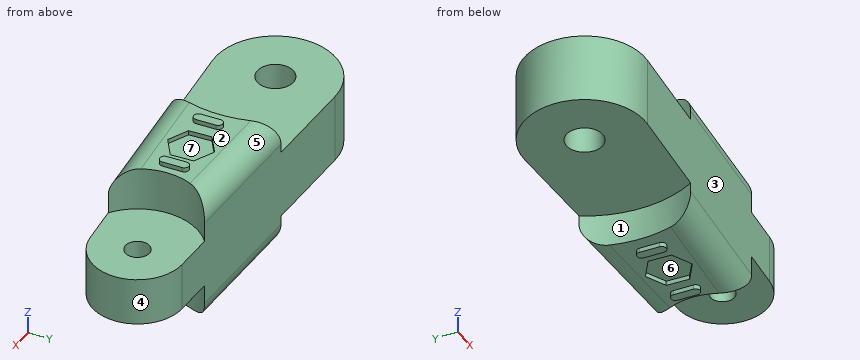
```python
from build123d import *

# Parameters (mm, degrees)
BOSS_EXTRUDE1_DEPTH    = 22.5
SKETCH2_R              = 37.5
SKETCH2_R_2            = 20
CUT_EXTRUDE1_DEPTH     = 11
FILLET1_R              = 8
SKETCH4_R              = 6
SKETCH4_R_2            = 4
CUT_EXTRUDE2_DEPTH     = 40
CUT_EXTRUDE3_DEPTH     = 1.5
BOSS_EXTRUDE2_DEPTH    = 1.5
SKETCH7_R              = 20
CUT_EXTRUDE4_DEPTH     = 3.5
BODY_MOVE_COPY7_ANGLE  = 178.232303169
BODY_MOVE_COPY8_ANGLE  = 1.26
BODY_MOVE_COPY9_ANGLE  = 1.26
BODY_MOVE_COPY10_ANGLE = 180


with BuildPart() as part:
    # Sketch1 → Boss-Extrude1 (new body, symmetric)
    with BuildSketch(Plane(origin=(0, 0, 0), x_dir=(1, 0, 0), z_dir=(0, 1, 0))):
        with BuildLine():
            Line((-91.135271219, -13.013928685), (-1.541618241, -19.940496814))
            ThreePointArc((-1.541618241, -19.940496814), (19.99534612, -0.431431984), (-0.680086883, 19.988433701))
            Line((-0.680086883, 19.988433701), (-90.489122701, 16.932769202))
            ThreePointArc((-90.489122701, 16.932769202), (-104.975567128, 2.265017913), (-91.135271219, -13.013928685))
        make_face()
    extrude(amount=BOSS_EXTRUDE1_DEPTH, both=True)

    # Sketch2 → Cut-Extrude1 (cut)
    with BuildSketch(Plane.XZ.offset(22.5)):
        Circle(SKETCH2_R)
        with Locations((-89.979057538, -1.941443926)):
            Circle(SKETCH2_R_2)
    cut_extrude1 = extrude(amount=-CUT_EXTRUDE1_DEPTH, mode=Mode.SUBTRACT)

    # Mirror1: Cut-Extrude1 across plane
    add(cut_extrude1.mirror(Plane(origin=(0, 0, 0), x_dir=(0, 0, 1), z_dir=(0, -1, 0))), mode=Mode.SUBTRACT)

    # Fillet1
    fillet1_edges = [part.edges().sort_by_distance(p)[0] for p in [
        (-55.557279033, -22.5, 15.764496148),
        (-54.825601141, -22.5, -18.1461856),
        (-54.825601141, 22.5, -18.1461856),
        (-55.557279033, 22.5, 15.764496148),
    ]]
    fillet(fillet1_edges, radius=FILLET1_R)

    # Sketch4 → Cut-Extrude2 (cut)
    with BuildSketch(Plane.XZ.offset(11.5)):
        Circle(SKETCH4_R)
        with Locations((-89.979057538, -1.941443926)):
            Circle(SKETCH4_R_2)
    extrude(amount=-CUT_EXTRUDE2_DEPTH, mode=Mode.SUBTRACT)

    # Sketch5 → Cut-Extrude3 (cut)
    with BuildSketch(Plane(origin=(0, 22.5, 0), x_dir=(1, 0, 0), z_dir=(0, 1, 0))):
        Polygon((-61.556626556, 4.801358237), (-61.398607028, -2.702531632), (-54.82103801, -6.31762764), (-48.401488521, -2.42883378), (-48.559508049, 5.075056088), (-55.137077066, 8.690152097), align=None)
    cut_extrude3 = extrude(amount=-CUT_EXTRUDE3_DEPTH, mode=Mode.SUBTRACT)

    # Sketch6 → Boss-Extrude2 (add)
    with BuildSketch(Plane(origin=(0, 22.5, 0), x_dir=(1, 0, 0), z_dir=(0, 1, 0))):
        with BuildLine():
            Line((-67.627696069, -1.919544043), (-67.627696069, 4.537052574))
            ThreePointArc((-67.627696069, 4.537052574), (-66.127696069, 6.037052574), (-64.627696069, 4.537052574))
            Line((-64.627696069, 4.537052574), (-64.627696069, -1.919544043))
            ThreePointArc((-64.627696069, -1.919544043), (-66.127696069, -3.419544043), (-67.627696069, -1.919544043))
        make_face()
        with BuildLine():
            Line((-44.491273974, -1.919544043), (-44.491273974, 4.537052574))
            ThreePointArc((-44.491273974, 4.537052574), (-42.991273974, 6.037052574), (-41.491273974, 4.537052574))
            Line((-41.491273974, 4.537052574), (-41.491273974, -1.919544043))
            ThreePointArc((-41.491273974, -1.919544043), (-42.991273974, -3.419544043), (-44.491273974, -1.919544043))
        make_face()
    boss_extrude2 = extrude(amount=BOSS_EXTRUDE2_DEPTH)

    # Mirror2: Cut-Extrude3, Boss-Extrude2 across plane
    add(cut_extrude3.mirror(Plane(origin=(0, 0, 0), x_dir=(0, 0, 1), z_dir=(0, -1, 0))), mode=Mode.SUBTRACT)
    add(boss_extrude2.mirror(Plane(origin=(0, 0, 0), x_dir=(0, 0, 1), z_dir=(0, -1, 0))))

    # Sketch7 → Cut-Extrude4 (cut)
    with BuildSketch(Plane.XZ.offset(11.5)):
        with Locations((-89.979057538, -1.941443926)):
            Circle(SKETCH7_R)
    cut_extrude4 = extrude(amount=-CUT_EXTRUDE4_DEPTH, mode=Mode.SUBTRACT)

    # Mirror3: Cut-Extrude4 across plane
    add(cut_extrude4.mirror(Plane.ZX), mode=Mode.SUBTRACT)


with BuildPart() as part_1:
    # Body-Move/Copy1: moved
    add(part.part.moved(Location((89.979057538, 0, 1.941443926))))


with BuildPart() as part_2:
    # Body-Move/Copy7: moved
    add(part_1.part.rotate(Axis((0, 0, 0), (-0.015427289, -0.70702263, 0.70702263)), BODY_MOVE_COPY7_ANGLE))


with BuildPart() as part_3:
    # Body-Move/Copy8: moved
    add(part_2.part.rotate(Axis((0, 0, 0), (0, 0, -1)), BODY_MOVE_COPY8_ANGLE))


with BuildPart() as part_4:
    # Body-Move/Copy9: moved
    add(part_3.part.rotate(Axis((0, 0, 0), (0, 0, 1)), BODY_MOVE_COPY9_ANGLE))


with BuildPart() as part_5:
    # Body-Move/Copy10: moved
    add(part_4.part.rotate(Axis((0, 0, 0), (1, 0, 0)), BODY_MOVE_COPY10_ANGLE))


solid = part_5.part
```
Verification items for the finished model (mm, model axes). Face numbers are marked on the shaded views. A direction names the side the tool comes from. Coordinates: 2 decimals unless noted, no trailing zeros. Loops run counter-clockwise (first coordinate to the right, second up) from the corner with the lowest first, then second, coordinate; pieces in that order, holes last. Notation, with made-up numbers: (69.25, 57.5) - (91.25, 57.5) arc R25 cw to (91.25, 75.5) - close; hole circle Ø10 at (-7, -4.5). An arc over 180 degrees is marked (long way). Answer as a JSON object with one key per item and string values.
(1) Scan lines: line 1 along Z through (x, y) = (-42, 4.5); line 2 along Z through (x, y) = (3.5, -6); line 3 along X through (y, z) = (0, 3.5). Record each from-to range of solid material in increasing order.
Response:
{"line 1": "z = -22.5 to 22.5", "line 2": "z = -8 to 8", "line 3": "x = -109.88 to -95.64, -84.32 to -4, 4 to 15"}
(2) Cross-section at A-A, the plane z = 1.5. Record the boundary of the cut face in (x, y), then the cut area to 3 significant figures.
Response:
{"outline": "(-89.31, 18) arc R20 ccw (long way) to (-88.43, -21.92) - (1.16, -14.95) arc R15 ccw to (0.5, 14.99) - close; hole circle Ø12 at (-89.98, -1.99); hole circle Ø8 at (0, 0)", "area": "3,970 mm²"}
(3) Cross-section at B-B, the plane z = 13. Record the boundary of the cut face in (x, y).
Response:
{"outline": "(-57.6, 16.94) arc R37.5 cw to (-56.8, -19.46) - (-12.03, -15.98) arc R20 cw to (-12.72, 15.43) - close"}
(4) Access from +Z, -Z, +X, -X, +Y, -Y to the whole of each face (thin tool, end or side, straight path). Record for the marked faces 5, 6 and 7.
Response:
{"face 5": "+Z, +X, +Y", "face 6": "-Z", "face 7": "+Z"}
(5) Mould release check, pull along Y, two halves, no side actions. Record for the marked faces 1, 2, 3 and 4: pulls with the +Y half, pulls with the -Y half, needs draft (parallel to the pull), parting line crosses it, or undercut.
Response:
{"face 1": "undercut", "face 2": "needs draft", "face 3": "pulls with the -Y half", "face 4": "parting line crosses it"}
(6) Cross-section at C-C, the plane x = -59.5. Record the boundary of the cut face in (y, z), then the cut area to 3 significant figures.
Response:
{"outline": "(-19.67, -11.5) - (17, -11.5) - (17, 11.5) - (-19.67, 11.5) - close", "area": "844 mm²"}
(7) Go/stop test with flat-tipped pins: pin 1 Ø3 at (x, y) = (-94.5, -12.5) entering from +Z; pin 2 Ø2 at (x, y) = (-37.5, 13.5) entering from +Z; pin 3 Ø6 at (x, z) = (-76.5, -11) entering from -Y; pin 4 Ø9.5 at (x, y) = (-89.98, -1.99) entering from -Z. Record where each tip stops, or that it passes through.
Response:
{"pin 1": "stops at z = 11.5", "pin 2": "stops at z = 21.29", "pin 3": "stops at y = -21.23", "pin 4": "passes through"}
